Design review of the part built by this model. Coordinates are the model's own, in mm. Face numbers are marked on the shaded views. A direction names the side the tool comes from. Give positions to 0.01 mm unless a question says otherwise; leave off trailing zeros. Order: outer loops, then holes, each group sorted by start corner. A loop starts at its lowest first (then second) coordinate and runs counter-clockwise, first axis right, second up. Notation, with made-up numbers: (36.5, -0.75) -> (79.5, -0.75) arc R15 cw to (79.5, 8.25) -> close; hole circle Ø11 at (83.25, -18). An arc over 180 degrees is marked (long way). One line per item, written item: value.
from build123d import *

# Parameters (mm, degrees)
EXTRUDE_1_DEPTH     = 33.5
SKETCH_6_R          = 6
CUT_EXTRUDE_2_DEPTH = 103.2
SKETCH_7_R          = 5.375
EXTRUDE_3_DEPTH     = 103.2
CUT_EXTRUDE_3_REACH = 84.471


with BuildPart() as part:
    # 草图1 → 凸台-拉伸1 (new body)
    with BuildSketch(Plane.XY):
        Polygon((51.6, -0.076277531), (51.6, 29.923722469), (20, 54.923722469), (-20, 54.923722469), (-51.6, 29.923722469), (-51.6, -0.076277531), align=None)
    extrude(amount=EXTRUDE_1_DEPTH)

    # 草图6 → 切除-拉伸2 (cut)
    with BuildSketch(Plane.ZY.offset(51.6)):
        with Locations((16.75, -0.076277531)):
            Circle(SKETCH_6_R)
    extrude(amount=-CUT_EXTRUDE_2_DEPTH, mode=Mode.SUBTRACT)

    # 草图7 → 凸台-拉伸3 (add)
    with BuildSketch(Plane.ZY.offset(51.6)):
        with Locations((5.375, -0.076277531)):
            Circle(SKETCH_7_R)
        with Locations((28.125, -0.076277531)):
            Circle(SKETCH_7_R)
    extrude(amount=-EXTRUDE_3_DEPTH)

    # 切除-拉伸3: up to this face of the body (flat: up to its plane)
    cut_extrude_3_end = Plane(part.part.faces().sort_by_distance((0, 24.324732157, 0))[0])
    # 草图8 → 切除-拉伸3 (cut, up to the picked face)
    with BuildSketch(Plane.XY.offset(33.5), mode=Mode.PRIVATE) as cut_extrude_3_sk1:
        Polygon((-46.6, -0.076277531), (-46.6, 24.923722469), (46.6, 24.923722469), (46.6, -0.076277531), (46.6, -12.111349377), (-46.6, -12.111349377), align=None)
    cut_extrude_3_tool1 = split(extrude(cut_extrude_3_sk1.sketch, amount=-CUT_EXTRUDE_3_REACH, mode=Mode.PRIVATE), bisect_by=cut_extrude_3_end, keep=Keep.BOTH, mode=Mode.PRIVATE)
    add(cut_extrude_3_tool1.solids().sort_by(Axis((0, 6.406187, 33.5), (0, 0, -1)))[0], mode=Mode.SUBTRACT)


solid = part.part
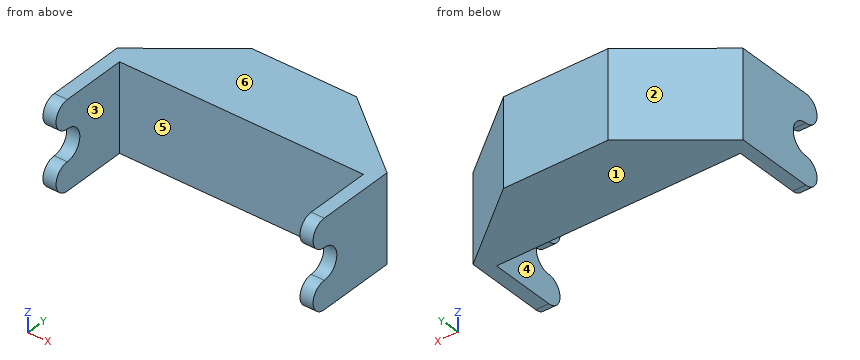
Item 1: Add section C-C on x = 13. Give the boundary of the cut face in (y, z), plus the area to 4 significant figures.
Returned:
outline: (24.92, 0) -> (54.92, 0) -> (54.92, 33.5) -> (24.92, 33.5) -> close
area: 1,005 mm²
Item 2: Draft analysis for pull direction X (two halves, no side actions). For the marked faces 1, 2, 3 and 4, state which applies: pulls with the +X half, pulls with the -X half, needs draft (parallel to the pull), parting line crosses it, or undercut.
Returned:
face 1: needs draft
face 2: pulls with the -X half
face 3: undercut
face 4: undercut
Item 3: Machinability: for the marked faces 5 and 6, which of the approach directions +Z, -Z, +X, -X, +Y, -Y give a long, thin tool a straight path to every point of the face, cutting with its end or side? Answer none if there is none.
Returned:
face 5: +Z, -Z, -Y
face 6: +Z, +X, -X, +Y, -Y
Item 4: Add section A-A on y = 22. Give the boundary of the cut face in (x, z), plus the area to 3 significant figures.
Returned:
outline: (-51.6, 0) -> (-46.6, 0) -> (-46.6, 33.5) -> (-51.6, 33.5) -> close; (46.6, 0) -> (51.6, 0) -> (51.6, 33.5) -> (46.6, 33.5) -> close
area: 335 mm²
Item 5: Add section B-B on z = 16.75. Give the boundary of the cut face in (x, y), plus the area to 3 significant figures.
Returned:
outline: (-51.6, 5.92) -> (-46.6, 5.92) -> (-46.6, 24.92) -> (46.6, 24.92) -> (46.6, 5.92) -> (51.6, 5.92) -> (51.6, 29.92) -> (20, 54.92) -> (-20, 54.92) -> (-51.6, 29.92) -> close
area: 2,500 mm²
Item 6: Add section D-D on y = 39.5. Give the boundary of the cut face in (x, z).
Returned:
outline: (-39.5, 0) -> (39.5, 0) -> (39.5, 33.5) -> (-39.5, 33.5) -> close
Item 7: To check wall thickness, follow line 1 along X through (y, z) = (6.5, 23); line 2 along Y through (x, z) = (0, 12); line 3 along Y through (x, z) = (46, 32). State the ranges of each line that lie inside material, in increasing order. Write a range as from..to.
Returned:
line 1: -51.6..-46.6, 46.6..51.6
line 2: 24.92..54.92
line 3: 24.92..34.35
Item 8: Clearance check with flat-ended pins moving along their axes: P1, Ø6, axis at y = 40.5, z = 5, coming from the -X side; P2, Ø2, axis at y = 33, z = 8, coming from the +X side; P3, Ø1, axis at y = 44, z = 25.5, coming from the +X side. State where each tip first meets the part, or that it passes through.
Returned:
P1: x = -42.02
P2: x = 48.98
P3: x = 34.44
